from build123d import *

# Parameters (mm, degrees)
F1_DEPTH = 1.95
F2_R     = 1.5
F3_DEPTH = 41
F4_W     = 29.75
F4_H     = 27
F5_DEPTH = 6.901
F6_SIZE  = 5


with BuildPart() as f1:
    # F0 (on Top) → F1 (new body)
    with BuildSketch(Plane.XY):
        Polygon((-7, 19.625), (-17, 19.625), (-17, 17.625), (-20.5, 17.625), (-20.5, -17.625), (-17, -17.625), (-17, -19.625), (-7, -19.625), (-7, -17.625), (7, -17.625), (7, -19.625), (17, -19.625), (17, -17.625), (20.5, -17.625), (20.5, 17.625), (17, 17.625), (17, 19.625), (7, 19.625), (7, 17.625), (-7, 17.625), align=None)
    extrude(amount=F1_DEPTH)

    # F2 (on face) → F3 (join, through all)
    with BuildSketch(Plane.YZ.offset(20.5)):
        with BuildLine():
            Line((-17.625, 1.95), (17.625, 1.95))
            ThreePointArc((17.625, 1.95), (0, 6.9), (-17.625, 1.95))
        make_face()
        with Locations((0, 3.5)):
            Circle(F2_R, mode=Mode.SUBTRACT)
    extrude(amount=-F3_DEPTH)

    # F4 (on face) → F5 (cut, through all)
    with BuildSketch(Plane(origin=(0, 0, 0), x_dir=(1, 0, 0), z_dir=(0, 0, -1))):
        Rectangle(F4_W, F4_H)
    extrude(amount=-F5_DEPTH, mode=Mode.SUBTRACT)

    # F6
    f6_edges = [f1.edges().sort_by_distance(p)[0] for p in [
        (14.875, -13.5, 2.045861),
        (-14.875, -13.5, 2.045861),
        (14.875, 13.5, 2.045861),
        (-14.875, 13.5, 2.045861),
    ]]
    chamfer(f6_edges, length=F6_SIZE)


solid = f1.part
Verification items for the finished model (mm, model axes). A direction names the side the tool comes from. Coordinates: 2 decimals unless noted, no trailing zeros. Write each loop counter-clockwise with the first axis right and the second up, starting at its lowest first coordinate (ties: lowest second). Pieces come first, ordered by that corner, then holes. Notation, with made-up numbers: (-0.75, 25) - (10.25, 25) arc R19 ccw to (10.25, 53) - close; hole circle Ø8 at (22.25, 60). An arc over 180 degrees is marked (long way). Answer as a JSON object with one key per item and string values.
(1) Cross-section at D-D on z = 0.5. Record the cut outline in (x, y) (3 decimals), plus the area to 3 significant figures.
Report:
{"outline": "(-20.5, -17.625) - (-17, -17.625) - (-17, -19.625) - (-7, -19.625) - (-7, -17.625) - (7, -17.625) - (7, -19.625) - (17, -19.625) - (17, -17.625) - (20.5, -17.625) - (20.5, 17.625) - (17, 17.625) - (17, 19.625) - (7, 19.625) - (7, 17.625) - (-7, 17.625) - (-7, 19.625) - (-17, 19.625) - (-17, 17.625) - (-20.5, 17.625) - close; hole (-14.875, -8.5) - (-9.875, -13.5) - (9.875, -13.5) - (14.875, -8.5) - (14.875, 8.5) - (9.875, 13.5) - (-9.875, 13.5) - (-14.875, 8.5) - close", "area": "772 mm^2"}
(2) Cross-section at C-C on y = 9.5. Record the cut outline in (x, z) (3 decimals), plus the area to 3 significant figures.
Report:
{"outline": "(-20.5, 0) - (-13.875, 0) - (-13.875, 5.54) - (-20.5, 5.54) - close; (13.875, 0) - (20.5, 0) - (20.5, 5.54) - (13.875, 5.54) - close", "area": "73.4 mm^2"}
(3) Tool access check on faces 1 (the flat face through (0, 13.5, 2)), 2 (the flat face through (-7, -19, 1)), 3 (the flat face through (-17, -19, 1)), 4 (the flat face through (-7, 19, 1)). Record the directions out of +Z, -Z, +X, -X, +Y, -Y that give a thin tool (end or side, any length) a straight path to the whole face; none if there is none.
Report:
{"face 1": "+Z, -Z", "face 2": "+Z, -Z, -Y", "face 3": "+Z, -Z, -X, -Y", "face 4": "+Z, -Z, +Y"}
(4) Cross-section at B-B on x = -2.5. Record the cut outline in (y, z) (3 decimals).
Report:
{"outline": "(-17.625, 0) - (-13.5, 0) - (-13.5, 4.092) arc R33.853 ccw to (-17.625, 1.95) - close; (13.5, 0) - (17.625, 0) - (17.625, 1.95) arc R33.853 ccw to (13.5, 4.092) - close"}
(5) Mould release check, pull along X, two halves, no side actions. Record for faces 5 (the flat face through (19, 17.625, 1)), 6 (the flat face through (-14.875, 2, 3)), 7 (the flat face through (20.5, 0, 1)), 8 (the flat face through (-12.34, 11.035, 2.221)): pulls with the +X half, pulls with the -X half, needs draft (parallel to the pull), parting line crosses it, or undercut.
Report:
{"face 5": "needs draft", "face 6": "undercut", "face 7": "pulls with the +X half", "face 8": "undercut"}
(6) Thickness scan on line 1 along X through (y, z) = (4, 2) (3 decimals); line 2 along Y through (x, z) = (8.5, 1.25) (3 decimals); line 3 along Z through (x, y) = (-16, 0). Record the ranges inside material, lowest first.
Report:
{"line 1": "-20.5 to -14.875, 14.875 to 20.5", "line 2": "-19.625 to -13.5, 13.5 to 19.625", "line 3": "0 to 2, 5 to 6.9"}
(7) Cross-section at A-A on y = 0. Record the cut outline in (x, z) (3 decimals), plus the area to 3 significant figures.
Report:
{"outline": "(-20.5, 0) - (-14.875, 0) - (-14.875, 2) - (-20.5, 2) - close; (-20.5, 5) - (-14.875, 5) - (-14.875, 6.9) - (-20.5, 6.9) - close; (14.875, 0) - (20.5, 0) - (20.5, 2) - (14.875, 2) - close; (14.875, 5) - (20.5, 5) - (20.5, 6.9) - (14.875, 6.9) - close", "area": "43.9 mm^2"}
(8) Gauge pin test, flat ends, axial feed: pin 1 Ø8 at (x, y) = (-1.5, -15.5) entering from +Z; pin 2 Ø1 at (x, y) = (-12, -19) entering from +Z; pin 3 Ø2 at (y, z) = (-19, 1) entering from +X; pin 4 Ø2.5 at (y, z) = (0, 3.5) entering from +X. Record the tip position at first contact, or that the pin passes through.
Report:
{"pin 1": "z = 4.09", "pin 2": "z = 1.95", "pin 3": "x = 17", "pin 4": "through"}
